Source: CAD feature listing. Evaluate the final solid. Frame: model axes, mm. Round coordinates to 2 decimals unless told otherwise and drop trailing zeros. Loops run counter-clockwise (first coordinate to the right, second up) from the corner with the lowest first, then second, coordinate; pieces in that order, holes last. Notation, with made-up numbers: (67, 72) - (110, 72) arc R15 cw to (110, 81) - close; hole circle Ø11 at (8.5, -27). An arc over 180 degrees is marked (long way). One line per question, with ' | ' between items.
from build123d import *

# Parameters (mm, degrees)
F1_DEPTH = 87.5
F3_R     = 1.5
F4_DEPTH = 28.751


with BuildPart() as f1:
    # F0 (on Top) → F1 (new body)
    with BuildSketch(Plane.XY):
        with BuildLine():
            ThreePointArc((0, -28.75), (20.3293199591, -20.3293199591), (28.75, 0))
            ThreePointArc((28.75, 0), (20.3293199591, 20.3293199591), (0, 28.75))
            Line((0, 28.75), (0, 27))
            ThreePointArc((0, 27), (19.091883092, 19.091883092), (27, 0))
            ThreePointArc((27, 0), (19.091883092, -19.091883092), (0, -27))
            Line((0, -27), (0, -28.75))
        make_face()
    extrude(amount=F1_DEPTH)

    # F3 (on Right) → F4 (cut, through all)
    with BuildSketch(Plane.YZ):
        with Locations((0, 65.625)):
            Circle(F3_R)
        with Locations((0, 21.875)):
            Circle(F3_R)
    extrude(amount=F4_DEPTH, mode=Mode.SUBTRACT)


solid = f1.part
1. Section query A-A, the plane x = 2.5. Return loops of the section in (y, z), plus the area to 3 significant figures.
Worked out:
outline: (-28.64, 0) - (-26.88, 0) - (-26.88, 87.5) - (-28.64, 87.5) - close; (26.88, 0) - (28.64, 0) - (28.64, 87.5) - (26.88, 87.5) - close | area: 307 mm2
2. Mould query, pull axis Y, two halves, no side actions, for faces 1 (the flat face through (0, 28, 43)), 2 (the cylindrical face through (27.84, -0.2, 23.36)). Classes: released by +Y, released by -Y, zero draft, split by the parting line, or undercut.
Worked out:
face 1: zero draft | face 2: undercut
3. Contact query for flat-ended pins moving along their axis: P1, Ø4, axis at x = 23, z = 23, coming from the -Y side; P2, Ø1, axis at x = 14, z = 23.5, coming from the -Y side; P3, Ø2, axis at x = 13.5, z = 56, coming from the +Y side. Output: stop coordinate, or through.
Worked out:
P1: stops at y = -19.64 | P2: stops at y = -25.38 | P3: stops at y = 25.89
4. Section query C-C, the plane x = 14. Return loops of the section in (y, z), plus the area to 3 significant figures.
Worked out:
outline: (-25.11, 0) - (-23.09, 0) - (-23.09, 87.5) - (-25.11, 87.5) - close; (23.09, 0) - (25.11, 0) - (25.11, 87.5) - (23.09, 87.5) - close | area: 354 mm2
5. Section query D-D, the plane y = -4. Return loops of the section in (x, z).
Worked out:
outline: (26.7, 0) - (28.47, 0) - (28.47, 87.5) - (26.7, 87.5) - close
6. Material intervals for probe 1 along Z at (x, y) = (27.6, 0) (3 decimals); probe 2 along Y at (x, z) = (18.75, 72); probe 3 along Y at (x, z) = (11, 56), sorted ascending.
Worked out:
probe 1: z = 0 to 20.375, 23.375 to 64.125, 67.125 to 87.5 | probe 2: y = -21.79 to -19.43, 19.43 to 21.79 | probe 3: y = -26.56 to -24.66, 24.66 to 26.56
7. Section query B-B, the plane z = 41. Return loops of the section in (x, y).
Worked out:
outline: (0, -28.75) arc R28.75 ccw to (0, 28.75) - (0, 27) arc R27 cw to (0, -27) - close
